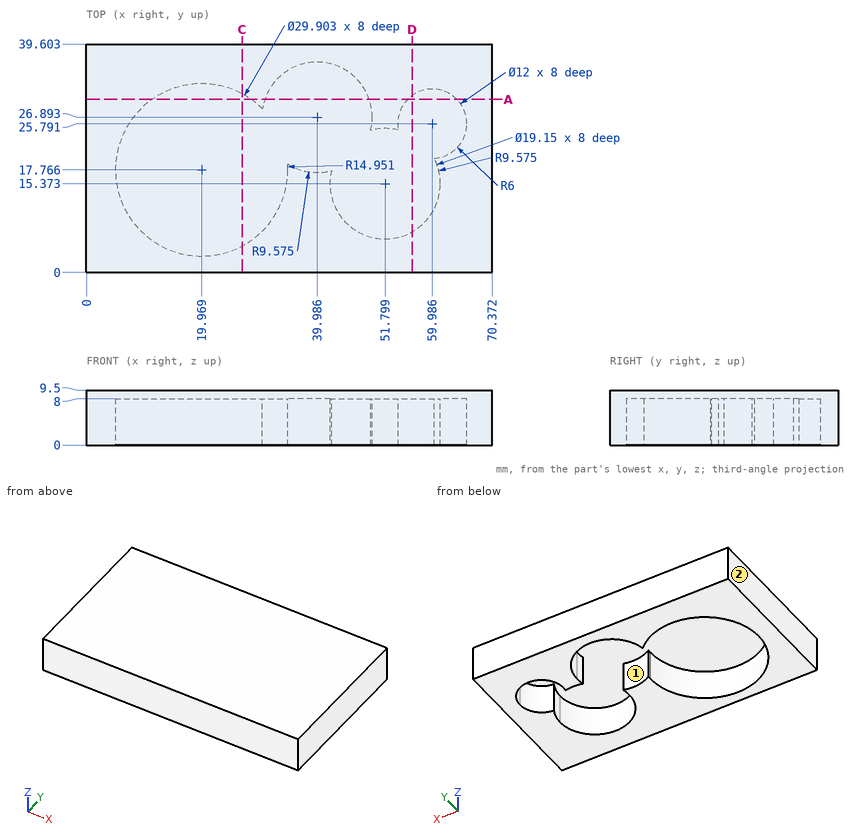
Input: dimensioned drawing with shaded views. Units: mm. Origin: part minimum x, y, z. A direction names the side the tool comes from. Coordinates: 2 decimals unless noted, no trailing zeros. Loops run counter-clockwise (first coordinate to the right, second up) from the corner with the lowest first, then second, coordinate; pieces in that order, holes last. Notation, with made-up numbers: (-1, 15.25) -> (33, 15.25) arc R37 ccw to (33, 53.25) -> close; hole circle Ø9 at (9, 43). An arc over 180 degrees is marked (long way). One line per item, written item: value. Start each with the question number.
Q1. Section query A-A, the plane y = 30. Return the cut outline in (x, z) (1 decimal).
Q2. Line query: line 1 along X through (y, z) = (30, 7.5) (1 decimal); line 2 along X through (y, z) = (16, 5.75) (1 decimal); line 3 along X through (y, z) = (29, 4.75) (1 decimal). Output: solid intervals per line, ascending.
Q3. Contact query for a flat-ended pin moving along its axis: P1, Ø4, axis at x = 22.5, y = 11, coming from the -Z side. Output: stop coordinate, or through.
Q4. Section query D-D, the plane x = 56.5. Return the cut outline in (y, z) (1 decimal), and give its area (3 significant figures).
Q5. Section query C-C, the plane x = 27. Return the cut outline in (y, z).
Q6. Set-up query: the marked faces 1 and 2. Return all of +Z, -Z, +X, -X, +Y, -Y with unobstructed straight access to the full face (end or side cutting, diameter ignored); none if empty.
Results:
1. outline: (0, 0) -> (11.4, 0) -> (11.4, 8) -> (28.6, 8) -> (28.6, 0) -> (30.9, 0) -> (30.9, 8) -> (49, 8) -> (49, 0) -> (55.7, 0) -> (55.7, 8) -> (64.3, 8) -> (64.3, 0) -> (70.4, 0) -> (70.4, 9.5) -> (0, 9.5) -> close
2. line 1: 0 to 11.4, 28.6 to 30.9, 49 to 55.7, 64.3 to 70.4
2. line 2: 0 to 5.1, 34.8 to 42.2, 61.4 to 70.4
2. line 3: 0 to 10.1, 29.8 to 30.6, 49.3 to 54.9, 65.1 to 70.4
3. P1: z = 8
4. outline: (0, 0) -> (7, 0) -> (7, 8) -> (30.7, 8) -> (30.7, 0) -> (39.6, 0) -> (39.6, 9.5) -> (0, 9.5) -> close
4. area: 187 mm^2
5. outline: (0, 0) -> (4.57, 0) -> (4.57, 8) -> (30.96, 8) -> (30.96, 0) -> (39.6, 0) -> (39.6, 9.5) -> (0, 9.5) -> close
6. face 1: -Z
6. face 2: +Z, -Z, -X, +Y, -Y
